Source: CAD feature listing. Evaluate the final solid. Frame: model axes, mm. Coordinates: 2 decimals unless noted, no trailing zeros. Order: outer loops, then holes, each group sorted by start corner. A loop starts at its lowest first (then second) coordinate and runs counter-clockwise, first axis right, second up.
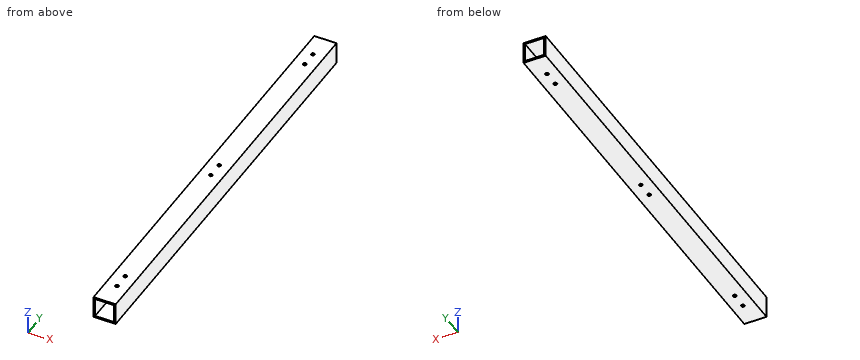
```python
from build123d import *

# Parameters (mm, degrees)
SKETCH1_W                        = 44.45
SKETCH1_H                        = 44.45
SKETCH1_W_2                      = 38.1
SKETCH1_H_2                      = 38.1
BOSS_EXTRUDE1_DEPTH              = 844.55
F_17_64_0_26563_DIAMETER_HOLE1_D = 6.747002


with BuildPart() as part:
    # Sketch1 → Boss-Extrude1 (new body)
    with BuildSketch(Plane(origin=(0, 0, 0), x_dir=(1, 0, 0), z_dir=(0, 1, 0))):
        with Locations((22.225, 22.225)):
            Rectangle(SKETCH1_W, SKETCH1_H)
        with Locations((22.225, 22.225)):
            Rectangle(SKETCH1_W_2, SKETCH1_H_2, mode=Mode.SUBTRACT)
    extrude(amount=BOSS_EXTRUDE1_DEPTH)

    # 17/64 (0.26563) Diameter Hole1 (through all)
    with Locations(Plane.XY):
        with Locations((22.225, 796.925), (22.225, 765.175), (22.225, 438.15), (22.225, 406.4), (22.225, 79.375), (22.225, 47.625)):
            Hole(F_17_64_0_26563_DIAMETER_HOLE1_D / 2)


solid = part.part
```
1. Section query A-A on x = 10. Return loops of the section in (y, z) (3 decimals).
Findings:
outline: (0, -44.45) - (844.55, -44.45) - (844.55, -41.275) - (0, -41.275) - close; (0, -3.175) - (844.55, -3.175) - (844.55, 0) - (0, 0) - close
2. Pin query (flat end, axial travel): P1, Ø8, axis at x = 22.225, y = 796.925, coming from the -Z side; P2, Ø5.5, axis at x = 22.225, y = 765.175, coming from the -Z side. Return the tip coordinate at first contact, or that it passes through.
Findings:
P1: stops at z = -44.45
P2: passes through
3. Ray query, line 1 (Z direction, x = 40, y = 87.5) (3 decimals); line 2 (X direction, y = 438.15, z = -0.95); line 3 (X direction, y = 117.5, z = -4) (3 decimals). Return the intervals inside material, ascending.
Findings:
line 1: z = -44.45 to -41.275, -3.175 to 0
line 2: x = 0 to 18.85, 25.6 to 44.45
line 3: x = 0 to 3.175, 41.275 to 44.45
4. Section query C-C on y = 639. Return loops of the section in (x, z) (3 decimals), plus the area to 3 significant figures.
Findings:
outline: (0, -44.45) - (44.45, -44.45) - (44.45, 0) - (0, 0) - close; hole (3.175, -41.275) - (41.275, -41.275) - (41.275, -3.175) - (3.175, -3.175) - close
area: 524 mm2
5. Section query B-B on z = -22. Return loops of the section in (x, y) (3 decimals), plus the area to 3 significant figures.
Findings:
outline: (0, 0) - (3.175, 0) - (3.175, 844.55) - (0, 844.55) - close; (41.275, 0) - (44.45, 0) - (44.45, 844.55) - (41.275, 844.55) - close
area: 5,360 mm2
